Verification items for the finished model (mm, model axes). A direction names the side the tool comes from. Coordinates: 2 decimals unless noted, no trailing zeros. Loops run counter-clockwise (first coordinate to the right, second up) from the corner with the lowest first, then second, coordinate; pieces in that order, holes last.
Q1. Sectioned sample at A-A (x = 8.75). Enter the section's corners in (y, z), then the cut area to 3 significant figures.
Q2. Sectioned sample at C-C (x = 15.75). Enter the section's corners in (y, z), then the cut area to 3 significant figures.
Q3. Go/stop test with flat-tipped pins: P1, Ø1.5, axis at x = 20.5, z = 6, coming from the -Y side; P2, Ø1.5, axis at x = 18.5, z = 5, coming from the -Y side; P3, Ø2.5, axis at x = 17.5, z = 4.5, coming from the +Y side. Record where each tip stops, or that it passes through.
Q4. Sectioned sample at B-B (y = -8.5). Enter the section's corners in (x, z).
Q5. Material ranges on probe 1 along Y at (x, z) = (17.25, 9.75); probe 2 along Y at (x, z) = (4, 2.5); probe 3 along X at (y, z) = (-13, 3.75), recorded low to high.
Q6. Mould release check, pull along X, two halves, no side actions. Record for faces 5 (the face through (18, -10.1, 5)), 6 (the face through (11, -10.3, 5.1)), 7 (the face through (6.524, 0.986, 4.368)): +X half, -X half, draft (parallel to the pull), parting line (faces both ways), or undercut.
Q7. Access from +Z, -Z, +X, -X, +Y, -Y to the whole of each face (thin tool, end or side, straight path). Record for faces 1 (the face through (18, 1.4, 5)), 2 (the face through (16.6, 0.64, 4.93)), 3 (the face through (7, -12.2, 5)), 4 (the face through (21, -6.2, 0.5)).
Q8. Sectioned sample at D-D (z = 1.5). Enter the section's corners in (x, y), then the cut area to 3 significant figures.
```python
from build123d import *

# Parameters (mm, degrees)
EXTRUDE_2_DEPTH     = 10
SKETCH_3_R          = 1.5
EXTRUDE_3_DEPTH     = 1.5
SKETCH_5_R          = 1.65
CUT_EXTRUDE_2_DEPTH = 3
FILLET_1_R          = 6
SKETCH_6_W          = 10
SKETCH_6_H          = 1
SKETCH_6_W_2        = 5
EXTRUDE_4_DEPTH     = 4
SKETCH_7_W          = 5.689599517
SKETCH_7_H          = 3.3
CUT_EXTRUDE_3_DEPTH = 0.5


with BuildPart() as part:
    # Эскиз2 → Бобышка-Вытянуть2 (new body)
    with BuildSketch(Plane.XY):
        Polygon((0, 0), (0, 2), (13, 2), (13, -0.1), (24, -0.1), (24, -2.1), (11, -2.1), (11, 0), align=None)
    extrude(amount=EXTRUDE_2_DEPTH)

    # Эскиз3 → Бобышка-Вытянуть3 (add)
    with BuildSketch(Plane(origin=(0, -0.1, 0), x_dir=(1, 0, 0), z_dir=(0, 1, 0))):
        with Locations((18.1, -5)):
            Circle(SKETCH_3_R)
    extrude(amount=EXTRUDE_3_DEPTH)

    # Эскиз5 → Вырез-Вытянуть2 (cut, through all)
    with BuildSketch(Plane.XZ):
        with Locations((5, 5)):
            Circle(SKETCH_5_R)
    extrude(amount=-CUT_EXTRUDE_2_DEPTH, mode=Mode.SUBTRACT)

    # Скругление1
    fillet_1_edges = [part.edges().sort_by_distance(p)[0] for p in [
        (24, -1.1, 10),
        (0, 1, 10),
    ]]
    fillet(fillet_1_edges, radius=FILLET_1_R)

    # Эскиз6 → Бобышка-Вытянуть4 (add)
    with BuildSketch(Plane(origin=(0, -2.1, 0), x_dir=(-1, 0, 0), z_dir=(0, -1, 0))):
        with Locations((-16, -0.5)):
            Rectangle(SKETCH_6_W, SKETCH_6_H)
        with Locations((-13.5, -9.5)):
            Rectangle(SKETCH_6_W_2, SKETCH_6_H)
    extrude(amount=EXTRUDE_4_DEPTH)

    # Эскиз7 → Вырез-Вытянуть3 (cut)
    with BuildSketch(Plane.XZ):
        with Locations((2.155200242, 5)):
            Rectangle(SKETCH_7_W, SKETCH_7_H)
    extrude(amount=-CUT_EXTRUDE_3_DEPTH, mode=Mode.SUBTRACT)

    # Зеркальное отражение1: part across plane


with BuildPart() as part_1:
    add(part.part)
    add(part.part.mirror(Plane.ZX.offset(-6.1)))


solid = part_1.part
```
Geometry check:
1. outline: (-14.2, 0) - (-12.2, 0) - (-12.2, 10) - (-14.2, 10) - close; (0, 0) - (2, 0) - (2, 10) - (0, 10) - close
1. area: 40.0 mm2
2. outline: (-12.1, 0) - (-0.1, 0) - (-0.1, 10) - (-12.1, 10) - close; hole (-10.1, 1) - (-2.1, 1) - (-2.1, 9) - (-10.1, 9) - close
2. area: 56.0 mm2
3. P1: stops at y = -12.1
3. P2: stops at y = -13.6
3. P3: stops at y = 1.4
4. outline: (11, 0) - (21, 0) - (21, 1) - (11, 1) - close; (11, 9) - (16, 9) - (16, 10) - (11, 10) - close
5. probe 1: y = -12.1 to -10.1, -2.1 to -0.1
5. probe 2: y = -14.2 to -12.2, 0 to 2
5. probe 3: x = 0 to 3.92, 6.08 to 13, 17.27 to 18.93
6. face 5: draft
6. face 6: -X half
6. face 7: undercut
7. face 1: +Z, -Z, +X, +Y
7. face 2: +Y
7. face 3: +Z, -Z, -X
7. face 4: +Z, -Z, +X
8. outline: (0, -14.2) - (13, -14.2) - (13, -12.1) - (24, -12.1) - (24, -10.1) - (11, -10.1) - (11, -12.2) - (0, -12.2) - close; (0, 0) - (11, 0) - (11, -2.1) - (24, -2.1) - (24, -0.1) - (13, -0.1) - (13, 2) - (0, 2) - close
8. area: 104 mm2
